```python
from build123d import *

# Parameters (mm, degrees)
F0_W     = 47.09104
F0_H     = 24.184491
F0_W_2   = 51.191684
F0_H_2   = 58.543412
F1_DEPTH = 72.644
F2_R     = 8.584943
F3_SIZE  = 5.08


with BuildPart() as f1:
    # F0 (on Front) → F1 (new body)
    with BuildSketch(Plane.XZ):
        with Locations((-13.492128, -38.009723)):
            Rectangle(F0_W, F0_H)
        Polygon((10.053392, -25.917478), (59.94251, -25.917478), (59.94251, -4.400743), (59.94251, 54.142669), (59.94251, 63.985944), (-58.487043, 63.985944), (-58.487043, -25.917478), (-37.037648, -25.917478), align=None)
        with Locations((85.538352, 24.870963)):
            Rectangle(F0_W_2, F0_H_2)
    extrude(amount=F1_DEPTH)

    # F2
    f2_edges = [f1.edges().sort_by_distance(p)[0] for p in [
        (85.538352, -72.644, -4.400743),
    ]]
    fillet(f2_edges, radius=F2_R)

    # F3
    f3_edges = [f1.edges().sort_by_distance(p)[0] for p in [
        (111.134194, -72.644, 29.163435),
        (85.538352, -72.644, 4.1842),
        (85.538352, -72.644, 54.142669),
        (59.94251, -72.644, -0.108271),
        (59.94251, -72.644, 59.064306),
        (59.94251, -72.644, -15.159111),
        (0.727734, -72.644, 63.985944),
        (34.997951, -72.644, -25.917478),
        (-58.487043, -72.644, 19.034233),
        (10.053392, -72.644, -38.009724),
        (-47.762346, -72.644, -25.917478),
        (-13.492128, -72.644, -50.101969),
        (-37.037648, -72.644, -38.009724),
    ]]
    chamfer(f3_edges, length=F3_SIZE)


solid = f1.part
```
Source: CAD feature listing. Evaluate the final solid. Frame: model axes, mm. A direction names the side the tool comes from. Coordinates: 2 decimals unless noted, no trailing zeros. Write each loop counter-clockwise with the first axis right and the second up, starting at its lowest first coordinate (ties: lowest second). Pieces come first, ordered by that corner, then holes. Notation, with made-up numbers: (81, 84) -> (102, 84) arc R21 ccw to (102, 115) -> close; hole circle Ø3 at (20, 61). An arc over 180 degrees is marked (long way). Return JSON: item names as keys, results as strings. Group by question number.
1) Section query A-A, the plane x = 14.5. Return loops of the section in (y, z), plus the area to 3 significant figures.
2) Ray query, line 1 along Z through (x, y) = (39, -33.5); line 2 along X through (y, z) = (-43.5, -38.5); line 3 along X through (y, z) = (-47.5, -13). Return the intervals inside material, ascending.
3) Section query B-B, the plane z = -19. Return loops of the section in (x, y), plus the area to 3 significant figures.
4) Set-up query: faces 1 (the face through (35, -33, -25.917)), 2 (the face through (82.604, -70.14, 51.567)), 3 (the face through (85, -33, 54.143)). Return all of +Z, -Z, +X, -X, +Y, -Y with unobstructed straight access to the full face (end or side cutting, diameter ignored); none if empty.
5) Contact query for flat-ended pins moving along their axis: P1, Ø5, axis at y = -32, z = 58.5, coming from the +X side; P2, Ø15, axis at x = 31.5, y = -26.5, coming from the -Z side; P3, Ø15.5, axis at x = 87, y = -49.5, coming from the +Z side. Output: stop coordinate, or through.
6) Section query C-C, the plane y = -17. Return loops of the section in (x, z), plus the area to 3 significant figures.
From the geometry:
{
 "1": {"outline": "(-72.64, -20.84) -> (-67.56, -25.92) -> (0, -25.92) -> (0, 63.99) -> (-67.56, 63.99) -> (-72.64, 58.91) -> close", "area": "6,510 mm²"},
 "2": {"line 1": "-25.92 to 63.99", "line 2": "-37.04 to 10.05", "line 3": "-58.49 to 59.94"},
 "3": {"outline": "(-58.49, -67.56) -> (-53.41, -72.64) -> (54.86, -72.64) -> (59.94, -67.56) -> (59.94, 0) -> (-58.49, 0) -> close", "area": "8,580 mm²"},
 "4": {"face 1": "-Z, +X, +Y, -Y", "face 2": "+Z, +X, -Y", "face 3": "+Z, +X, +Y, -Y"},
 "5": {"P1": "x = 59.94", "P2": "z = -25.92", "P3": "z = 54.14"},
 "6": {"outline": "(-58.49, -25.92) -> (-37.04, -25.92) -> (-37.04, -50.1) -> (10.05, -50.1) -> (10.05, -25.92) -> (59.94, -25.92) -> (59.94, -4.4) -> (106.05, -4.4) -> (111.13, 0.68) -> (111.13, 54.14) -> (59.94, 54.14) -> (59.94, 63.99) -> (-58.49, 63.99) -> close", "area": "14,800 mm²"}
}
